Drawing for the job (mm, zero at the part's lowest x, y, z). A direction names the side the tool comes from. Give positions to 0.01 mm unless a question says otherwise; leave off trailing zeros. Order: outer loops, then holes, each group sorted by start corner. A loop starts at its lowest first (then second) coordinate and runs counter-clockwise, first axis right, second up. Notation, with made-up numbers: M 72,58 L 85,58 A27 cw 85,74 Z; hole C -3.5,57.25 d8. An arc over 180 degrees is marked long. Answer as a JSON object with one key per item and string values.
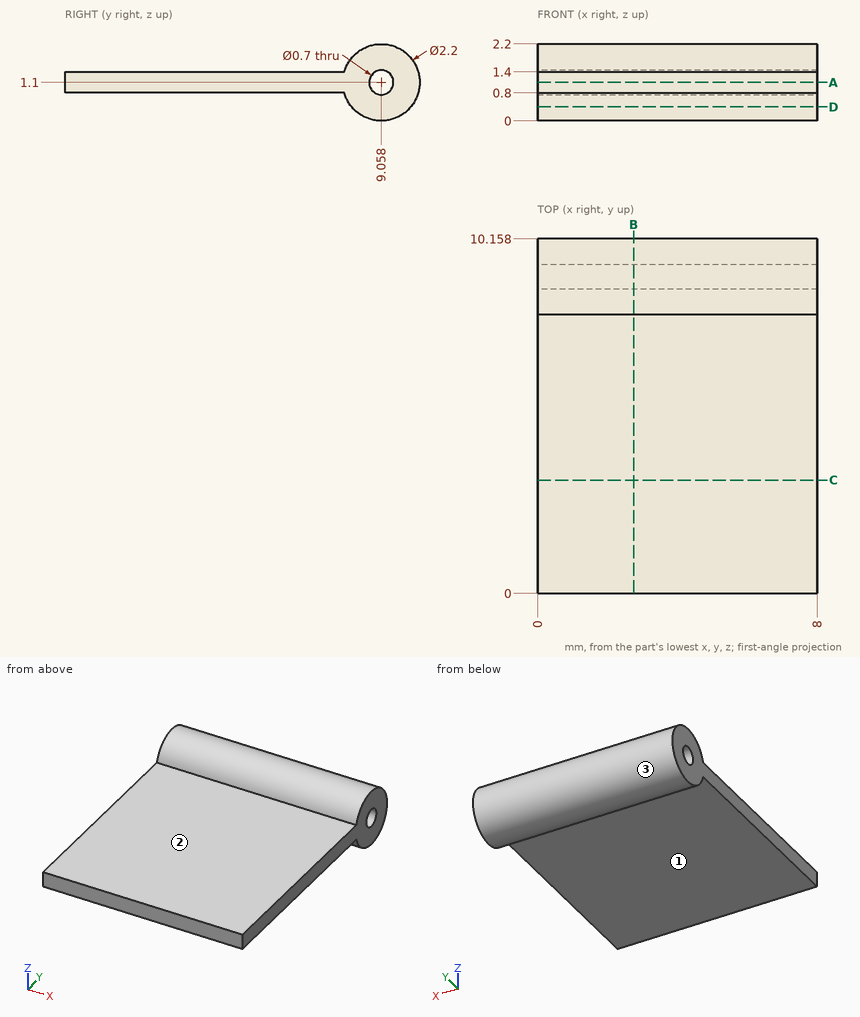
1. Cut at C-C on y = 3.25. Give the cut face in (x, z).
Worked answers:
{"outline": "M 0,0.8 L 8,0.8 L 8,1.4 L 0,1.4 Z"}
2. Cut at B-B on x = 2.75. Give the cut face in (y, z).
Worked answers:
{"outline": "M 0,0.8 L 8,0.8 A1.1 ccw long 8,1.4 L 0,1.4 Z; hole C 9.06,1.1 d0.7"}
3. Which spindle directions (+Z, -Z, +X, -X, +Y, -Y) get a long thin tool onto all of the face, cutting with end or side? Do the marked faces 1, 2 and 3. Say none if no direction does.
Worked answers:
{"face 1": "-Z, +X, -X, -Y", "face 2": "+Z, +X, -X, -Y", "face 3": "+X, -X"}
4. Cut at A-A on z = 1.1. Give the cut face in (x, y).
Worked answers:
{"outline": "M 0,0 L 8,0 L 8,8.71 L 0,8.71 Z; M 0,9.41 L 8,9.41 L 8,10.16 L 0,10.16 Z"}
5. Probe line 1 along Y through (x, z) = (5, 1.05) (1 decimal); line 2 along Z through (x, y) = (7.5, 2.5); line 3 along Y through (x, z) = (2.75, 1.35) (1 decimal). List the from-to ranges inside material, lowest first.
Worked answers:
{"line 1": "y = 0 to 8.7, 9.4 to 10.2", "line 2": "z = 0.8 to 1.4", "line 3": "y = 0 to 8.8, 9.3 to 10.1"}
6. Cut at D-D on z = 0.4. Give the cut face in (x, y).
Worked answers:
{"outline": "M 0,8.21 L 8,8.21 L 8,9.91 L 0,9.91 Z"}
7. Pin check, flat tip, straight feed: P1, Ø4, axis at x = 2.5, y = 3, coming from the +Z side. Stop position of the tip, or through.
Worked answers:
{"P1": "stops at z = 1.4"}
